Input: part model. Units: mm. Frame: model coordinates. Face numbers are marked on the shaded views. A direction names the side the tool comes from. Round coordinates to 2 decimals unless told otherwise and drop trailing zeros. Loops run counter-clockwise (first coordinate to the right, second up) from the corner with the lowest first, then second, coordinate; pieces in that order, holes last. Notation, with made-up numbers: M 37,47 L 91,47 A24 ccw 91,74 Z; hole C -33,64 d5. An arc over 180 degrees is marked long. Put each result on its own line as item: value. Start each with the question number.
1) Line query: probe 1 along Y at (x, z) = (150, 8); probe 2 along X at (y, z) = (-90.5, 7.75); probe 3 along Z at (x, y) = (154, -116). Output: solid intervals per line, ascending.
2) Section C-C on y = -98. Output: boundary loops of the cut face in (x, z), plus the area to 3 significant figures.
3) Section B-B on z = -1.25. Output: boundary loops of the cut face in (x, y), plus the area to 3 significant figures.
4) Pin query (flat end, axial travel): pin 1 (12 mm diameter, centred on x = 192.5, y = -123, fed in from -Z); pin 2 (24 mm diameter, centred on x = 160.5, y = -94, fed in from -Z). Return the tip coordinate at first contact, or that it passes through.
5) Reachability of the marked faces 5 and 6 from +Z, -Z, +X, -X, +Y, -Y: full face, straight path, thin tool, end or side. Return the list, or none.
6) Draft query along X for the marked faces 1, 2, 3 and 4. Return one class per face: +X half, -X half, draft (parallel to the pull), parting line (faces both ways), or undercut.
7) Section A-A on x = 162. Output: boundary loops of the cut face in (y, z), plus the area to 3 significant figures.
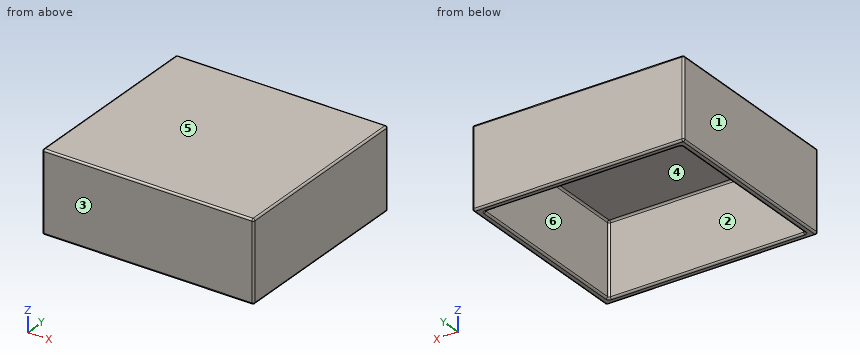
from build123d import *

# Parameters (mm, degrees)
SKETCH003_W   = 57.8
SKETCH003_H   = 53.16
PAD002_DEPTH  = 2
SKETCH004_W   = 57.8
SKETCH004_H   = 53.16
SKETCH004_W_2 = 53.8
SKETCH004_H_2 = 49.16
PAD003_DEPTH  = 20
FILLET_R      = 0.5


with BuildPart() as part:
    # Sketch003 (on Face23 of ShapeBinder001) → Pad002 (new body)
    with BuildSketch(Plane.XY.offset(10.4)):
        with Locations((171.25, -106.07)):
            Rectangle(SKETCH003_W, SKETCH003_H)
    extrude(amount=PAD002_DEPTH)

    # Sketch004 (on Face5 of Pad002) → Pad003 (join)
    with BuildSketch(Plane(origin=(0, 0, 10.4), x_dir=(1, 0, 0), z_dir=(0, 0, -1))):
        with Locations((171.25, 106.07)):
            Rectangle(SKETCH004_W, SKETCH004_H)
        with Locations((171.25, 106.07)):
            Rectangle(SKETCH004_W_2, SKETCH004_H_2, mode=Mode.SUBTRACT)
    extrude(amount=PAD003_DEPTH)

    # Fillet
    fillet_edges = [part.edges().sort_by_distance(p)[0] for p in [
        (171.25, -132.65, -9.6),
        (142.35, -106.07, -9.6),
        (171.25, -79.49, -9.6),
        (200.15, -106.07, -9.6),
        (171.25, -130.65, -9.6),
        (144.35, -106.07, -9.6),
        (171.25, -81.49, -9.6),
        (198.15, -106.07, -9.6),
        (198.15, -130.65, 0.4),
        (144.35, -130.65, 0.4),
        (171.25, -130.65, 10.4),
        (144.35, -81.49, 0.4),
        (144.35, -106.07, 10.4),
        (198.15, -81.49, 0.4),
        (171.25, -81.49, 10.4),
        (198.15, -106.07, 10.4),
        (200.15, -79.49, 1.4),
        (142.35, -79.49, 1.4),
        (171.25, -79.49, 12.4),
        (142.35, -106.07, 12.4),
        (171.25, -132.65, 12.4),
        (200.15, -106.07, 12.4),
        (200.15, -132.65, 1.4),
        (142.35, -132.65, 1.4),
    ]]
    fillet(fillet_edges, radius=FILLET_R)


solid = part.part
Geometry results:
1. probe 1: y = -132.65 to -130.65, -81.49 to -79.49
1. probe 2: x = 142.35 to 144.35, 198.15 to 200.15
1. probe 3: z = 10.4 to 12.4
2. outline: M 142.35,-9.1 A0.5 ccw 142.85,-9.6 L 143.85,-9.6 A0.5 ccw 144.35,-9.1 L 144.35,9.9 A0.5 cw 144.85,10.4 L 197.65,10.4 A0.5 cw 198.15,9.9 L 198.15,-9.1 A0.5 ccw 198.65,-9.6 L 199.65,-9.6 A0.5 ccw 200.15,-9.1 L 200.15,11.9 A0.5 ccw 199.65,12.4 L 142.85,12.4 A0.5 ccw 142.35,11.9 Z
2. area: 195 mm²
3. outline: M 142.35,-132.15 A0.5 ccw 142.85,-132.65 L 199.65,-132.65 A0.5 ccw 200.15,-132.15 L 200.15,-79.99 A0.5 ccw 199.65,-79.49 L 142.85,-79.49 A0.5 ccw 142.35,-79.99 Z; hole M 144.35,-130.15 A0.5 ccw 144.85,-130.65 L 197.65,-130.65 A0.5 ccw 198.15,-130.15 L 198.15,-81.99 A0.5 ccw 197.65,-81.49 L 144.85,-81.49 A0.5 ccw 144.35,-81.99 Z
3. area: 428 mm²
4. pin 1: stops at z = -9.58
4. pin 2: stops at z = 10.4
5. face 5: +Z, +X, -X, +Y, -Y
5. face 6: -Z
6. face 1: -X half
6. face 2: undercut
6. face 3: draft
6. face 4: undercut
7. outline: M -132.65,-9.1 A0.5 ccw -132.15,-9.6 L -131.15,-9.6 A0.5 ccw -130.65,-9.1 L -130.65,9.9 A0.5 cw -130.15,10.4 L -81.99,10.4 A0.5 cw -81.49,9.9 L -81.49,-9.1 A0.5 ccw -80.99,-9.6 L -79.99,-9.6 A0.5 ccw -79.49,-9.1 L -79.49,11.9 A0.5 ccw -79.99,12.4 L -132.15,12.4 A0.5 ccw -132.65,11.9 Z
7. area: 186 mm²
